Input: part model. Units: mm. Frame: model coordinates. Round coordinates to 2 decimals unless told otherwise and drop trailing zeros. Loops run counter-clockwise (first coordinate to the right, second up) from the corner with the lowest first, then second, coordinate; pieces in that order, holes last. Notation, with made-up numbers: (-13, 46.5) -> (27, 46.5) arc R15 ccw to (27, 65.5) -> close; hole circle Ø1 at (17.5, 56.5). An arc over 180 degrees is marked (long way). One line per question, with ' | ' between items. Start each with the question number.
Q1. Cut plane A-A on z = 2.5. Return loops of the section in (x, y).
Q2. Cut plane B-B on x = 92. Return loops of the section in (y, z), and give its area (3 significant figures).
Q3. Contact query for flat-ended pins moving along their axis: P1, Ø1.5, axis at y = 79, z = 2, coming from the +X side; P2, Ø1, axis at y = 55, z = 1.5, coming from the +X side. Output: stop coordinate, or through.
Q4. Material intervals for L1, parallel to X at y = 77, z = 1.75; L2, parallel to Y at x = -100.5, z = 2; L3, parallel to Y at x = -19.5, z = 1, sorted ascending.
Q5. Cut plane C-C on y = -13. Return loops of the section in (x, z).
from build123d import *

# Parameters (mm, degrees)
SKETCH1_W           = 244
SKETCH1_H           = 180
BOSS_EXTRUDE1_DEPTH = 3
CUT_EXTRUDE1_DEPTH  = 3
CUT_EXTRUDE2_DEPTH  = 3


with BuildPart() as part:
    # Sketch1 → Boss-Extrude1 (new body)
    with BuildSketch(Plane.XY):
        Rectangle(SKETCH1_W, SKETCH1_H)
    extrude(amount=BOSS_EXTRUDE1_DEPTH)

    # Sketch2 → Cut-Extrude1 (cut)
    with BuildSketch(Plane.XY.offset(3)):
        Polygon((122, 90), (63.514454678, -90), (122, -90), align=None)
    extrude(amount=-CUT_EXTRUDE1_DEPTH, mode=Mode.SUBTRACT)

    # Sketch3 → Cut-Extrude2 (cut)
    with BuildSketch(Plane.XY.offset(3)):
        with BuildLine():
            Line((-80, 83), (-80, 73))
            ThreePointArc((-80, 73), (-82, 71), (-84, 73))
            Line((-84, 73), (-84, 83))
            ThreePointArc((-84, 83), (-82, 85), (-80, 83))
        make_face()
        with BuildLine():
            Line((-17, 83), (-17, 73))
            ThreePointArc((-17, 73), (-19, 71), (-21, 73))
            Line((-21, 73), (-21, 83))
            ThreePointArc((-21, 83), (-19, 85), (-17, 83))
        make_face()
        with BuildLine():
            Line((45, 83), (45, 73))
            ThreePointArc((45, 73), (43, 71), (41, 73))
            Line((41, 73), (41, 83))
            ThreePointArc((41, 83), (43, 85), (45, 83))
        make_face()
        with BuildLine():
            Line((-112, 2), (-102, 2))
            ThreePointArc((-102, 2), (-100, 0), (-102, -2))
            Line((-102, -2), (-112, -2))
            ThreePointArc((-112, -2), (-114, 0), (-112, 2))
        make_face()
        with BuildLine():
            Line((-112, -80.5), (-102, -80.5))
            ThreePointArc((-102, -80.5), (-100, -82.5), (-102, -84.5))
            Line((-102, -84.5), (-112, -84.5))
            ThreePointArc((-112, -84.5), (-114, -82.5), (-112, -80.5))
        make_face()
    extrude(amount=-CUT_EXTRUDE2_DEPTH, mode=Mode.SUBTRACT)


solid = part.part
Results:
1) outline: (-122, -90) -> (63.51, -90) -> (122, 90) -> (-122, 90) -> close; hole (-112, -84.5) -> (-102, -84.5) arc R2 ccw to (-102, -80.5) -> (-112, -80.5) arc R2 ccw to start; hole (-112, -2) -> (-102, -2) arc R2 ccw to (-102, 2) -> (-112, 2) arc R2 ccw to start; hole (-84, 73) arc R2 ccw to (-80, 73) -> (-80, 83) arc R2 ccw to (-84, 83) -> close; hole (-21, 73) arc R2 ccw to (-17, 73) -> (-17, 83) arc R2 ccw to (-21, 83) -> close; hole (41, 73) arc R2 ccw to (45, 73) -> (45, 83) arc R2 ccw to (41, 83) -> close
2) outline: (-2.33, 0) -> (90, 0) -> (90, 3) -> (-2.33, 3) -> close | area: 277 mm^2
3) P1: x = 118.67 | P2: x = 110.79
4) L1: -122 to -84, -80 to -21, -17 to 41, 45 to 117.78 | L2: -90 to -83.82, -81.18 to -1.32, 1.32 to 90 | L3: -90 to 71.06, 84.94 to 90
5) outline: (-122, 0) -> (88.53, 0) -> (88.53, 3) -> (-122, 3) -> close
